For this review, take the finished solid that the model builds, in its own axes (mm). Face numbers are marked on the shaded views. A direction names the side the tool comes from. Give positions to 0.01 mm unless a question says otherwise; leave off trailing zeros. Loops run counter-clockwise (first coordinate to the right, second up) from the corner with the lowest first, then second, coordinate; pieces in that order, holes last. Notation, with made-up numbers: (44, -34) - (51, -34) arc R30 cw to (51, 5) - close; hole circle Ø4 at (22.5, 57.5). An arc over 180 degrees is marked (long way). Answer in a Markdown table with one row per item.
```python
from build123d import *

# Parameters (mm, degrees)
F0_W     = 84.236942
F0_H     = 59.479135
F1_DEPTH = 3.048
F2_W     = 84.236942
F2_H     = 59.479135
F2_W_2   = 79.999916
F2_H_2   = 54.874644
F3_DEPTH = 14.986
F4_R     = 5.08
F5_W     = 39.552113
F5_H     = 43.175208
F6_DEPTH = 25.4


with BuildPart() as f1:
    # F0 (on Top) → F1 (new body)
    with BuildSketch(Plane.XY):
        with Locations((-1.28318, -2.792804)):
            Rectangle(F0_W, F0_H)
    extrude(amount=F1_DEPTH)

    # F2 (on face) → F3 (join)
    with BuildSketch(Plane(origin=(0, 0, 0), x_dir=(1, 0, 0), z_dir=(0, 0, -1))):
        with Locations((-1.28318, 2.792804)):
            Rectangle(F2_W, F2_H)
        with Locations((-1.188636, 2.879139)):
            Rectangle(F2_W_2, F2_H_2, mode=Mode.SUBTRACT)
    extrude(amount=F3_DEPTH)

    # F4
    f4_edges = [f1.edges().sort_by_distance(p)[0] for p in [
        (-43.401651, -2.792805, 3.048),
        (-1.28318, -32.532372, 3.048),
        (40.835291, -2.792805, 3.048),
        (-1.28318, 26.946763, 3.048),
    ]]
    fillet(f4_edges, radius=F4_R)

    # F5 (on face) → F6 (cut)
    with BuildSketch(Plane.XY.offset(3.048)):
        with Locations((-15.171708, -2.792801)):
            Rectangle(F5_W, F5_H)
    extrude(amount=-F6_DEPTH, mode=Mode.SUBTRACT)


solid = f1.part
```
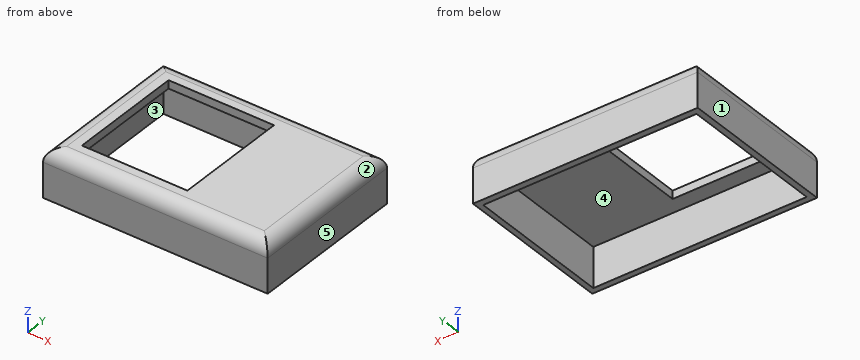
1. Clearance check with flat-ended pins moving along their axes: pin 1 (3.5 mm diameter, centred on y = -9.5, z = 2, fed in from -X); pin 2 (3.5 mm diameter, centred on y = -0.5, z = 1, fed in from +X); pin 3 (6 mm diameter, centred on x = 0, y = -7, fed in from -Z); pin 4 (2.5 mm diameter, centred on x = -6, z = 1, fed in from -Y). State where each tip first meets the part, or that it passes through.
Values:
| item | result |
|---|---|
| pin 1 | stops at x = -42.86 |
| pin 2 | stops at x = 40.67 |
| pin 3 | passes through |
| pin 4 | stops at y = -32.21 |
2. For the marked faces 4 and 5, list the 3-axis set-ups (+Z, -Z, +X, -X, +Y, -Y) from which the entire face can be reached by the end or side of a thin tool; tool diameter is ignored.
Values:
| item | result |
|---|---|
| face 4 | -Z |
| face 5 | +Z, -Z, +X, +Y, -Y |
3. We need section B-B, the plane z = -3.25. Give the boundary of the cut face in (x, y).
Values:
| item | result |
|---|---|
| outline | (-43.4, -32.53) - (40.84, -32.53) - (40.84, 26.95) - (-43.4, 26.95) - close; hole (-41.19, -30.32) - (38.81, -30.32) - (38.81, 24.56) - (-41.19, 24.56) - close |
4. We need section C-C, the plane y = 10.5. Give the boundary of the cut face in (x, z), and give its area (3 significant figures).
Values:
| item | result |
|---|---|
| outline | (-43.4, -14.99) - (-41.19, -14.99) - (-41.19, 0) - (-34.95, 0) - (-34.95, 3.05) - (-38.32, 3.05) arc R5.08 ccw to (-43.4, -2.03) - close; (4.6, 0) - (38.81, 0) - (38.81, -14.99) - (40.84, -14.99) - (40.84, -2.03) arc R5.08 ccw to (35.76, 3.05) - (4.6, 3.05) - close |
| area | 189 mm^2 |
5. Mouldability with a two-part tool opening along X and no side actions: class the marked faces 1, 2 and 3 as released by +X, released by -X, zero draft, split by the parting line, or undercut.
Values:
| item | result |
|---|---|
| face 1 | released by -X |
| face 2 | released by +X |
| face 3 | undercut |
6. We need section A-A, the plane x = -24.5. Give the boundary of the cut face in (y, z).
Values:
| item | result |
|---|---|
| outline | (-32.53, -14.99) - (-30.32, -14.99) - (-30.32, 0) - (-24.38, 0) - (-24.38, 3.05) - (-27.45, 3.05) arc R5.08 ccw to (-32.53, -2.03) - close; (18.79, 0) - (24.56, 0) - (24.56, -14.99) - (26.95, -14.99) - (26.95, -2.03) arc R5.08 ccw to (21.87, 3.05) - (18.79, 3.05) - close |
7. We need section D-D, the plane x = 28. Give the boundary of the cut face in (y, z).
Values:
| item | result |
|---|---|
| outline | (-32.53, -14.99) - (-30.32, -14.99) - (-30.32, 0) - (24.56, 0) - (24.56, -14.99) - (26.95, -14.99) - (26.95, -2.03) arc R5.08 ccw to (21.87, 3.05) - (-27.45, 3.05) arc R5.08 ccw to (-32.53, -2.03) - close |
8. Wall thickness on line 1 (Y direction, x = -13, z = -7.75); line 2 (X direction, y = 2, z = -10.5); line 3 (Z direction, x = 12.5, y = -24): over which ranges is each line inside the solid? List them lowest first. Write a range as [from, to].
Values:
| item | result |
|---|---|
| line 1 | y = [-32.53, -30.32], [24.56, 26.95] |
| line 2 | x = [-43.4, -41.19], [38.81, 40.84] |
| line 3 | z = [0, 3.05] |
